Could you check a few things on this model? Use its own coordinates, in mm. Face numbers are marked on the shaded views. Round coordinates to 2 decimals unless told otherwise and drop trailing zeros. Loops run counter-clockwise (first coordinate to the right, second up) from the corner with the lowest first, then second, coordinate; pieces in that order, holes last. Notation, with made-up numbers: M 7.5,66 L 18.5,66 A7 cw 18.5,70 Z; hole C 17.25,32 d9. An arc over 180 degrees is marked long. Answer in a Markdown table with one row per item.
Autodesk Inventor part; units mm, degrees
ref_plane "YZ Plane" through (0, 0, 0) normal (1, 0, 0) x (0, 1, 0)
ref_plane "XZ Plane" through (0, 0, 0) normal (0, 1, 0) x (-1, 0, 0)
ref_plane "XY Plane" through (0, 0, 0) normal (0, 0, 1) x (1, 0, 0)
sketch "Sketch1" plane through (0, 0, 0) normal (0, 1, 0) x (-1, 0, 0)
  line L0 (0, 0) -> (12, 0)
  line L1 (12, 0) -> (12, -26)
  line L2 (12, -26) -> (0, -26)
  line L3 (0, -26) -> (0, 0)
  dimension "d0" = 12
  dimension "d1" = 26
extrude "Extrusion1" add sketch "Sketch1" along normal blind 1
sketch "Sketch2" plane through (0, 1, 0) normal (0, 1, 0) x (1, 0, 0)
  line L0 (-8.4967, 0) -> (-6.4967, 0)
  line L1 (-6.4967, 0) -> (-6.4967, 2)
  line L2 (-6.4967, 2) -> (-8.4967, 2)
  line L3 (-8.4967, 2) -> (-8.4967, 0)
  line L4 (-5.264, 0) -> (-3.264, 0)
  line L5 (-3.264, 0) -> (-3.264, 2)
  line L6 (-3.264, 2) -> (-5.264, 2)
  line L7 (-5.264, 2) -> (-5.264, 0)
  line L8 (0, 26) -> (-12, 26)
  line L9 (-8.4967, 26) -> (-6.4967, 26)
  line L10 (-6.4967, 26) -> (-6.4967, 24)
  line L11 (-6.4967, 24) -> (-8.4967, 24)
  line L12 (-8.4967, 24) -> (-8.4967, 26)
  line L13 (-5.264, 24) -> (-3.264, 24)
  line L14 (-3.264, 24) -> (-3.264, 26)
  line L15 (-3.264, 26) -> (-5.264, 26)
  line L16 (-5.264, 26) -> (-5.264, 24)
  line L17 (-6, 10.9212) -> (-3.3419, 10.9212)
  line L18 (-3.3419, 10.9212) -> (-3.3419, 16.5565)
  line L19 (-3.3419, 16.5565) -> (-6, 16.5565)
  line L20 (-6, 16.5565) -> (-6, 10.9212)
  point P0 (0, 0)
  dimension "d4" = 2
  dimension "d5" = 2
  dimension "d6" = 2
  dimension "d7" = 2
  dimension "d8" = 2
extrude "Extrusion2" add sketch "Sketch2" along normal blind 1.5
sketch "Sketch3" plane through (0, 2.5, 0) normal (0, 1, 0) x (1, 0, 0)
  line L0 (-7.7977, 0.5679) -> (-7.2977, 0.5679)
  line L1 (-7.2977, 0.5679) -> (-7.2977, 1.0679)
  line L2 (-7.2977, 1.0679) -> (-7.7977, 1.0679)
  line L3 (-7.7977, 1.0679) -> (-7.7977, 0.5679)
  line L4 (-4.303, 0.5679) -> (-3.803, 0.5679)
  line L5 (-3.803, 0.5679) -> (-3.803, 1.0679)
  line L6 (-3.803, 1.0679) -> (-4.303, 1.0679)
  line L7 (-4.303, 1.0679) -> (-4.303, 0.5679)
  line L8 (-7.7977, 24.5946) -> (-7.2977, 24.5946)
  line L9 (-7.2977, 24.5946) -> (-7.2977, 25.0946)
  line L10 (-7.2977, 25.0946) -> (-7.7977, 25.0946)
  line L11 (-7.7977, 25.0946) -> (-7.7977, 24.5946)
  line L12 (-4.303, 24.5946) -> (-3.803, 24.5946)
  line L13 (-3.803, 24.5946) -> (-3.803, 25.0946)
  line L14 (-3.803, 25.0946) -> (-4.303, 25.0946)
  line L15 (-4.303, 25.0946) -> (-4.303, 24.5946)
  point P0 (0, 0)
  dimension "d11" = 0.5
  dimension "d12" = 0.5
  dimension "d13" = 0.5
  dimension "d14" = 0.5
  dimension "d15" = 0.5
  dimension "d16" = 0.5
extrude "Extrusion3" add sketch "Sketch3" along normal blind 2
sketch "Sketch4" plane through (0, 1, 0) normal (0, 1, 0) x (1, 0, 0)
  line L0 (-6.7275, 22.8918) -> (-4.7275, 22.8918)
  line L1 (-4.7275, 22.8918) -> (-4.7275, 21.8918)
  line L2 (-4.7275, 21.8918) -> (-6.7275, 21.8918)
  line L3 (-6.7275, 21.8918) -> (-6.7275, 22.8918)
  line L4 (-6.7275, 20.1179) -> (-4.7275, 20.1179)
  line L5 (-4.7275, 20.1179) -> (-4.7275, 21.1179)
  line L6 (-4.7275, 21.1179) -> (-6.7275, 21.1179)
  line L7 (-6.7275, 21.1179) -> (-6.7275, 20.1179)
  line L8 (-4.7275, 4.0841) -> (-6.7275, 4.0841)
  line L9 (-6.7275, 4.0841) -> (-6.7275, 3.0841)
  line L10 (-6.7275, 3.0841) -> (-4.7275, 3.0841)
  line L11 (-4.7275, 3.0841) -> (-4.7275, 4.0841)
  line L12 (-6.7275, 4.8554) -> (-4.7275, 4.8554)
  line L13 (-4.7275, 4.8554) -> (-4.7275, 5.8554)
  line L14 (-4.7275, 5.8554) -> (-6.7275, 5.8554)
  line L15 (-6.7275, 5.8554) -> (-6.7275, 4.8554)
  point P0 (0, 0)
  dimension "d19" = 2
  dimension "d20" = 1
  dimension "d21" = 2
  dimension "d22" = 1
  dimension "d23" = 2
  dimension "d24" = 1
  dimension "d25" = 2
  dimension "d26" = 1
extrude "Extrusion4" add sketch "Sketch4" along normal blind 1
sketch "Sketch5" plane through (0, 1, 0) normal (0, 1, 0) x (1, 0, 0)
  line L0 (-10.8338, 5.7882) -> (-9.3922, 5.7882)
  line L1 (-9.3922, 5.7882) -> (-9.3922, 3.0841)
  line L2 (-9.3922, 3.0841) -> (-10.8338, 3.0841)
  line L3 (-10.8338, 3.0841) -> (-10.8338, 5.7882)
  line L4 (-10.8338, 22.8302) -> (-9.3922, 22.8302)
  line L5 (-9.3922, 22.8302) -> (-9.3922, 20.0926)
  line L6 (-9.3922, 20.0926) -> (-10.8338, 20.0926)
  line L7 (-10.8338, 20.0926) -> (-10.8338, 22.8302)
  point P0 (0, 0)
extrude "Extrusion5" add sketch "Sketch5" along normal blind 0.7
sketch "Sketch6" plane through (0, 1, 0) normal (0, 1, 0) x (1, 0, 0)
  point P0 (0, 0)
sketch "Sketch7" plane through (0, 1, 0) normal (0, 1, 0) x (1, 0, 0)
  line L0 (-3.3419, 16.5565) -> (-3.3419, 10.9212)
  line L1 (-3.3419, 16.0376) -> (-1.9546, 16.0376)
  line L2 (-1.9546, 16.0376) -> (-1.9546, 15.4008)
  line L3 (-1.9546, 15.4008) -> (-3.3419, 15.4008)
  line L4 (-3.3419, 15.4008) -> (-3.3419, 16.0376)
  line L5 (-3.3419, 14.1925) -> (-1.9546, 14.1925)
  line L6 (-1.9546, 14.1925) -> (-1.9546, 13.5115)
  line L7 (-1.9546, 13.5115) -> (-3.3419, 13.5115)
  line L8 (-3.3419, 13.5115) -> (-3.3419, 14.1925)
  line L9 (-3.3419, 12.1636) -> (-1.9546, 12.1636)
  line L10 (-1.9546, 12.1636) -> (-1.9546, 11.5661)
  line L11 (-1.9546, 11.5661) -> (-3.3419, 11.5661)
  line L12 (-3.3419, 11.5661) -> (-3.3419, 12.1636)
  line L13 (-6, 10.9212) -> (-6, 16.5565)
  line L14 (-6, 14.8304) -> (-7.4823, 14.8304)
  line L15 (-7.4823, 14.8304) -> (-7.4823, 12.8104)
  line L16 (-7.4823, 12.8104) -> (-6, 12.8104)
  line L17 (-6, 12.8104) -> (-6, 14.8304)
  point P0 (0, 0)
extrude "Extrusion6" add sketch "Sketch7" along normal blind 0.7
properties part number "dc to dc"
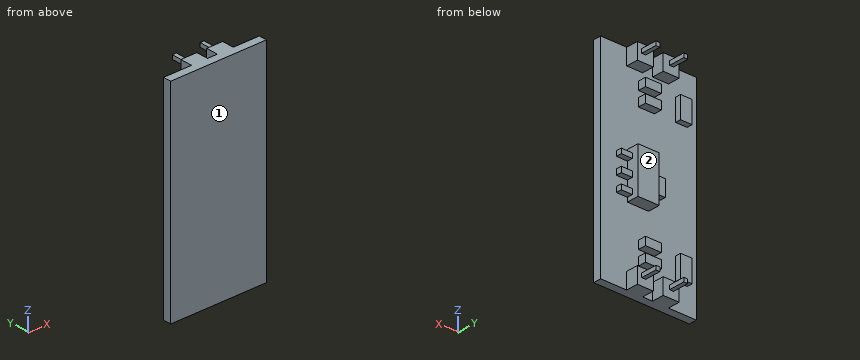
1) Will these pins go through, and if not, where does the flat tip stop? P1, Ø0.6, axis at x = -2.5, y = 1.5, coming from the -Z side; P2, Ø1.5, axis at x = -7, z = -19.5, coming from the +Y side; P3, Ø2, axis at x = -7, z = -25.5, coming from the +Y side; P4, Ø0.8, axis at y = 2, z = -25, coming from the -X side.
Computed:
| item | result |
|---|---|
| P1 | stops at z = -16.04 |
| P2 | stops at y = 2 |
| P3 | stops at y = 4.5 |
| P4 | stops at x = -8.5 |
2) I want a section at D-D, the plane z = -13.75. Please give me the cut outline in (x, y).
Computed:
| item | result |
|---|---|
| outline | M -12,0 L 0,0 L 0,1 L -1.95,1 L -1.95,1.7 L -3.34,1.7 L -3.34,2.5 L -6,2.5 L -6,1.7 L -7.48,1.7 L -7.48,1 L -12,1 Z |
3) I want a section at A-A, the plane y = 3.8. Please give me the cut outline in (x, z), plus the area to 3 significant figures.
Computed:
| item | result |
|---|---|
| outline | M -7.8,-25.09 L -7.3,-25.09 L -7.3,-24.59 L -7.8,-24.59 Z; M -7.8,-1.07 L -7.3,-1.07 L -7.3,-0.57 L -7.8,-0.57 Z; M -4.3,-25.09 L -3.8,-25.09 L -3.8,-24.59 L -4.3,-24.59 Z; M -4.3,-1.07 L -3.8,-1.07 L -3.8,-0.57 L -4.3,-0.57 Z |
| area | 1.00 mm² |
4) I need wall thicknesses on line 1 (Z direction, x = -5, y = 2.1); line 2 (Z direction, x = -3, y = 1.6); line 3 (Y direction, x = -7, z = -5). Which ranges of each line are inside material? Lowest first, please.
Computed:
| item | result |
|---|---|
| line 1 | z = -26 to -24, -16.56 to -10.92, -2 to 0 |
| line 2 | z = -16.04 to -15.4, -14.19 to -13.51, -12.16 to -11.57 |
| line 3 | y = 0 to 1 |
5) If we mould it in two halves opening along Z, with no side actions, what happens to the marked faces 1 and 2? For each: released by +Z, released by -Z, zero draft, split by the parting line, or undercut.
Computed:
| item | result |
|---|---|
| face 1 | zero draft |
| face 2 | undercut |
6) I want a section at B-B, the plane x = -10. Please give me the cut outline in (y, z), plus the area to 3 significant figures.
Computed:
| item | result |
|---|---|
| outline | M 0,-26 L 1,-26 L 1,-22.83 L 1.7,-22.83 L 1.7,-20.09 L 1,-20.09 L 1,-5.79 L 1.7,-5.79 L 1.7,-3.08 L 1,-3.08 L 1,0 L 0,0 Z |
| area | 29.8 mm² |
7) I want a section at C-C, the plane y = 2.25. Please give me the cut outline in (x, z), plus the area to 3 significant figures.
Computed:
| item | result |
|---|---|
| outline | M -8.5,-26 L -6.5,-26 L -6.5,-24 L -8.5,-24 Z; M -8.5,-2 L -6.5,-2 L -6.5,0 L -8.5,0 Z; M -6,-16.56 L -3.34,-16.56 L -3.34,-10.92 L -6,-10.92 Z; M -5.26,-26 L -3.26,-26 L -3.26,-24 L -5.26,-24 Z; M -5.26,-2 L -3.26,-2 L -3.26,0 L -5.26,0 Z |
| area | 31.0 mm² |
